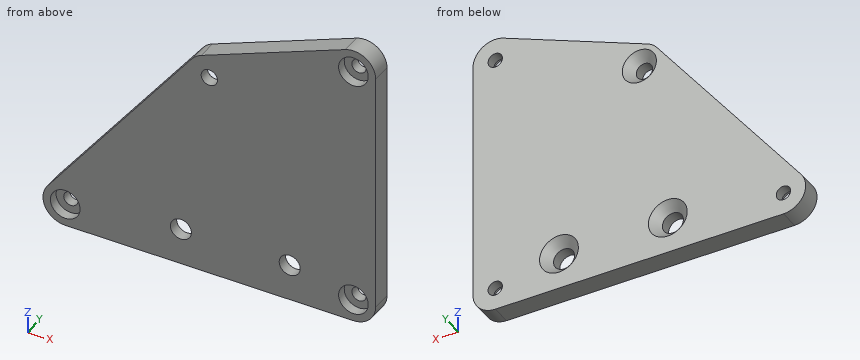
from build123d import *

# Parameters (mm, degrees)
SKETCH1_R           = 3
SKETCH1_R_2         = 2.125
SKETCH1_R_3         = 1.65
BOSS_EXTRUDE1_DEPTH = 4
SKETCH1_3_R         = 3
SKETCH1_3_R_2       = 1.45
BOSS_EXTRUDE2_DEPTH = 2
CHAMFER1_SIZE       = 1.8


with BuildPart() as part:
    # Sketch1 → Boss-Extrude1 (new body)
    with BuildSketch(Plane(origin=(0, 0, 0), x_dir=(1, 0, 0), z_dir=(0, 1, 0))):
        with BuildLine():
            Line((29.125, 29), (-29.125, 29))
            ThreePointArc((-29.125, 29), (-33.166733686, 26.478481442), (-32.678997817, 21.739728362))
            Line((-32.678997817, 21.739728362), (-3.553997817, -15.760271638))
            ThreePointArc((-3.553997817, -15.760271638), (-2.699104035, -16.600671799), (-1.652658398, -17.185537029))
            Line((-1.652658398, -17.185537029), (27.472341602, -28.685537029))
            ThreePointArc((27.472341602, -28.685537029), (31.656110153, -28.22068292), (33.625, -24.5))
            Line((33.625, -24.5), (33.625, 24.5))
            ThreePointArc((33.625, 24.5), (32.306980515, 27.681980515), (29.125, 29))
        make_face()
        with Locations(Location((29.125, 24.5, 0), (0, 0, 270))):
            Circle(SKETCH1_R, mode=Mode.SUBTRACT)
        with Locations(Location((-29.125, 24.5, 0), (0, 0, 270))):
            Circle(SKETCH1_R, mode=Mode.SUBTRACT)
        with Locations(Location((29.125, -24.5, 0), (0, 0, 270))):
            Circle(SKETCH1_R, mode=Mode.SUBTRACT)
        with Locations(Location((16.25, 21.625, 0), (0, 0, 270))):
            Circle(SKETCH1_R_2, mode=Mode.SUBTRACT)
        with Locations(Location((-5.75, 21.625, 0), (0, 0, 270))):
            Circle(SKETCH1_R_2, mode=Mode.SUBTRACT)
        with Locations(Location((0, -13, 0), (0, 0, 270))):
            Circle(SKETCH1_R_3, mode=Mode.SUBTRACT)
    extrude(amount=-BOSS_EXTRUDE1_DEPTH)

    # Sketch1_3 → Boss-Extrude2 (add)
    # profile 1 of 3: a face of its own
    with BuildSketch(Plane(origin=(0, 0, 0), x_dir=(1, 0, 0), z_dir=(0, 1, 0))):
        with Locations(Location((29.125, -24.5, 0), (0, 0, 270))):
            Circle(SKETCH1_3_R)
        with Locations(Location((29.125, -24.5, 0), (0, 0, 270))):
            Circle(SKETCH1_3_R_2, mode=Mode.SUBTRACT)
    # profile 2 of 3: a face of its own
    with BuildSketch(Plane(origin=(0, 0, 0), x_dir=(1, 0, 0), z_dir=(0, 1, 0))):
        with Locations(Location((-29.125, 24.5, 0), (0, 0, 270))):
            Circle(SKETCH1_3_R)
        with Locations(Location((-29.125, 24.5, 0), (0, 0, 270))):
            Circle(SKETCH1_3_R_2, mode=Mode.SUBTRACT)
    # profile 3 of 3: a face of its own
    with BuildSketch(Plane(origin=(0, 0, 0), x_dir=(1, 0, 0), z_dir=(0, 1, 0))):
        with Locations(Location((29.125, 24.5, 0), (0, 0, 270))):
            Circle(SKETCH1_3_R)
        with Locations(Location((29.125, 24.5, 0), (0, 0, 270))):
            Circle(SKETCH1_3_R_2, mode=Mode.SUBTRACT)
    extrude(amount=-BOSS_EXTRUDE2_DEPTH)

    # Chamfer1
    chamfer1_edges = [part.edges().sort_by_distance(p)[0] for p in [
        (0, 0, 11.35),
        (-5.75, 0, -23.75),
        (16.25, 0, -23.75),
    ]]
    chamfer(chamfer1_edges, length=CHAMFER1_SIZE)


solid = part.part
Part model, mm, in its own coordinate system. Coordinates: 2 decimals unless noted, no trailing zeros. Order: outer loops, then holes, each group sorted by start corner. A loop starts at its lowest first (then second) coordinate and runs counter-clockwise, first axis right, second up. Notation, with made-up numbers: (24.5, 48) - (29.5, 48) arc R16 ccw to (29.5, 76) - close; hole circle Ø5 at (-37, 29.5). An arc over 180 degrees is marked (long way). Use CSV: the item, a comma, the result in double quotes.
Item 1: Saw through at D-D on z = -11.5. Give the cut face in (x, y) (3 decimals).
Solved:
outline,"(-24.726, -4) - (33.625, -4) - (33.625, 0) - (-24.726, 0) - close"
Item 2: Probe probe 1 along X at (y, z) = (-3.2, -24.5) (3 decimals); probe 2 along X at (y, z) = (-0.5, -24.5) (3 decimals); probe 3 along Z at (x, y) = (28, -0.8). List the from-to ranges inside material, lowest first.
Solved:
probe 1,"x = -33.625 to -32.125, -26.125 to 26.125, 32.125 to 33.625"
probe 2,"x = -33.625 to -30.575, -27.675 to -7.611, -3.889 to 14.389, 18.111 to 27.675, 30.575 to 33.625"
probe 3,"z = -29 to -25.41, -23.59 to 23.59, 25.41 to 28.86"
Item 3: Saw through at C-C on z = 13. Give the cut face in (x, y) (3 decimals).
Solved:
outline,"(-5.698, -4) - (-1.65, -4) - (-1.65, -1.8) - (-3.45, 0) - (-5.698, 0) - close; (1.65, -4) - (33.625, -4) - (33.625, 0) - (3.45, 0) - (1.65, -1.8) - close"
Item 4: Saw through at A-A on y = -3.35. Give the cut face in (x, z) (3 decimals).
Solved:
outline,"(-32.679, -21.74) arc R4.5 ccw to (-29.125, -29) - (29.125, -29) arc R4.5 ccw to (33.625, -24.5) - (33.625, 24.5) arc R4.5 ccw to (27.472, 28.686) - (-1.653, 17.186) arc R4.5 ccw to (-3.554, 15.76) - close; hole circle Ø6 at (-29.125, -24.5); hole circle Ø4.25 at (-5.75, -21.625); hole circle Ø3.3 at (0, 13); hole circle Ø4.25 at (16.25, -21.625); hole circle Ø6 at (29.125, -24.5); hole circle Ø6 at (29.125, 24.5)"
Item 5: Saw through at B-B on x = 16.25. Give the cut face in (y, z).
Solved:
outline,"(-4, -29) - (0, -29) - (0, -25.55) - (-1.8, -23.75) - (-4, -23.75) - close; (-4, -19.5) - (-1.8, -19.5) - (0, -17.7) - (0, 24.25) - (-4, 24.25) - close"
Item 6: Drop flat-ended pins along their axis: P1, Ø4, axis at x = 29.125, z = 24.5, coming from the -Y side; P2, Ø1, axis at x = 24.5, y = -0.5, coming from the +Z side; P3, Ø4, axis at x = 0, z = 13, coming from the +Y side. Give the stop position or say it passes through.
Solved:
P1,"stops at y = -2"
P2,"stops at z = 27.71"
P3,"stops at y = -1.45"
